Design review of the part built by this model. Coordinates are the model's own, in mm. A direction names the side the tool comes from. Round coordinates to 2 decimals unless told otherwise and drop trailing zeros. Loops run counter-clockwise (first coordinate to the right, second up) from the corner with the lowest first, then second, coordinate; pieces in that order, holes last. Notation, with made-up numbers: M 70,-37 L 119,-37 A28 cw 119,-13 Z; hole C 24.25,34 d8. An arc over 180 degrees is marked long. Use a Markdown table: item, result.
Autodesk Inventor part; units mm, degrees
ref_plane "YZ Plane" through (0, 0, 0) normal (1, 0, 0) x (0, 1, 0)
ref_plane "XZ Plane" through (0, 0, 0) normal (0, 1, 0) x (-1, 0, 0)
ref_plane "XY Plane" through (0, 0, 0) normal (0, 0, 1) x (1, 0, 0)
sketch "Sketch2" plane through (0, 0, 0) normal (0, 0, 1) x (1, 0, 0)
  line L0 (0, 0) -> (5, 0)
  line L1 (5, 0) -> (5, 13)
  line L2 (0, 9.9166) -> (0, 0)
  line L3 (5, 13) -> (70, 13)
  line L4 (70, 13) -> (70, 18)
  line L5 (70, 18) -> (0, 18)
  line L6 (0, 18) -> (0, 9.9166)
  dimension "d9" = 5
  dimension "d10" = 65
  dimension "d11" = 13
  dimension "d16" = 5
extrude "Extrusion2" add sketch "Sketch2" along normal blind 10
fillet "Fillet1" radius 15 1 edges at (0, 18, 5)
fillet "Fillet2" radius 10 1 edges at (5, 13, 5)
properties part number "zweef-01"
1. Take a section at A-A on x = 59. Give the boundary of the cut face in (y, z).
Check values:
| item | result |
|---|---|
| outline | M 13,0 L 18,0 L 18,10 L 13,10 Z |
2. Machinability: for faces 1 (the face through (42, 13, 5)), 2 (the face through (43, 18, 5)), which of the approach directions +Z, -Z, +X, -X, +Y, -Y give a long, thin tool a straight path to every point of the face, cutting with its end or side? Answer none if there is none.
Check values:
| item | result |
|---|---|
| face 1 | +Z, -Z, +X, -Y |
| face 2 | +Z, -Z, +X, -X, +Y |
3. Insertion check: pin 1 (4 mm diameter, centred on x = 45.5, z = 2, fed in from -Y); pin 2 (1 mm diameter, centred on y = 11, z = 6.5, fed in from -X); pin 3 (2.5 mm diameter, centred on y = 2, z = 7.5, fed in from +X). Each pin has a flat end and moves straight along its axis. Give the tip position at first contact, or say it passes through.
Check values:
| item | result |
|---|---|
| pin 1 | stops at y = 13 |
| pin 2 | stops at x = 2.01 |
| pin 3 | stops at x = 5 |
4. Wall thickness on line 1 along Y through (x, z) = (46.5, 5.5); line 2 along X through (y, z) = (3, 1.5); line 3 along X through (y, z) = (11.5, 8): over which ranges is each line inside the solid? List them lowest first. Write a range as from..to.
Check values:
| item | result |
|---|---|
| line 1 | y = 13..18 |
| line 2 | x = 0..5 |
| line 3 | x = 2.64..9.73 |
